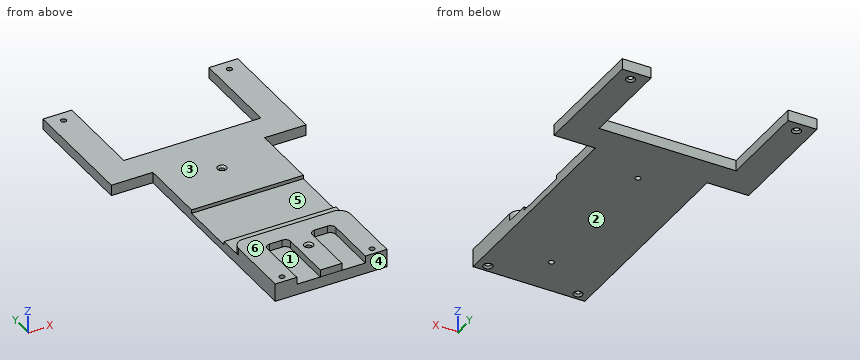
```python
from build123d import *

# Parameters (mm, degrees)
SKETCH_R        = 1.5
PAD_DEPTH       = 6
SKETCH001_R     = 1.5
PAD001_DEPTH    = 4
SKETCH002_R     = 1.5
POCKET_DEPTH    = 10
CHAMFER_SIZE    = 1
SKETCH003_W     = 100
SKETCH003_H     = 32
POCKET001_DEPTH = 2


with BuildPart() as part:
    # Sketch → Pad (new body)
    with BuildSketch(Plane.XY):
        Polygon((-38, 29), (38, 29), (38, 80), (54, 80), (54, 13), (31, 13), (31, -107), (-31, -107), (-31, 13), (-54, 13), (-54, 80), (-38, 80), align=None)
        Circle(SKETCH_R, mode=Mode.SUBTRACT)
        with Locations((0, -85)):
            Circle(SKETCH_R, mode=Mode.SUBTRACT)
        with Locations((46, 74)):
            Circle(SKETCH_R, mode=Mode.SUBTRACT)
        with Locations((-46, 74)):
            Circle(SKETCH_R, mode=Mode.SUBTRACT)
    extrude(amount=PAD_DEPTH)

    # Sketch001 (on Face18 of Pad) → Pad001 (join)
    with BuildSketch(Plane.XY.offset(6)):
        with BuildLine():
            Line((31, -71), (31, -107))
            Line((19, -107), (31, -107))
            Line((19, -78.000015), (19, -107))
            ThreePointArc((19, -78.000015), (18.12132, -75.878696), (16.000001, -75.000016))
            Line((8.999999, -75.000016), (16.000001, -75.000016))
            ThreePointArc((8.999999, -75.000016), (6.878678, -75.878697), (6, -78.000019))
            Line((6, -107.000009), (6, -78.000019))
            Line((-6, -107.000009), (6, -107.000009))
            Line((-6, -78.000019), (-6, -107.000009))
            ThreePointArc((-6, -78.000019), (-6.878676, -75.878693), (-8.999999, -75.000009))
            Line((-16.000001, -75.000009), (-8.999999, -75.000009))
            ThreePointArc((-16.000001, -75.000009), (-18.12132, -75.878689), (-19, -78.000009))
            Line((-19, -107), (-19, -78.000009))
            Line((-31, -107), (-19, -107))
            Line((-31, -107), (-31, -71))
            ThreePointArc((-25, -65), (-29.242641, -66.757359), (-31, -71))
            Line((-25, -65), (25, -65))
            ThreePointArc((31, -71), (29.242641, -66.757359), (25, -65))
        make_face()
        with Locations((0, -85)):
            Circle(SKETCH001_R, mode=Mode.SUBTRACT)
    extrude(amount=PAD001_DEPTH)

    # Sketch002 (on Face30 of Pad001) → Pocket (cut)
    with BuildSketch(Plane.XY.offset(10)):
        with Locations((-25, -103)):
            Circle(SKETCH002_R)
        with Locations((25, -103)):
            Circle(SKETCH002_R)
    extrude(amount=-POCKET_DEPTH, mode=Mode.SUBTRACT)

    # Chamfer
    chamfer_edges = [part.edges().sort_by_distance(p)[0] for p in [
        (23.5, -103, 0),
        (-26.5, -103, 0),
        (-47.5, 74, 0),
        (44.5, 74, 0),
        (-1.5, -85, 10),
        (-1.5, 0, 6),
    ]]
    chamfer(chamfer_edges, length=CHAMFER_SIZE)

    # Sketch003 (on Face21 of Chamfer) → Pocket001 (cut)
    with BuildSketch(Plane.XY.offset(6)):
        with Locations((0, -41)):
            Rectangle(SKETCH003_W, SKETCH003_H)
    extrude(amount=-POCKET001_DEPTH, mode=Mode.SUBTRACT)


solid = part.part
```
Work out the finished part from the listing and answer in its coordinate system (mm). Face numbers are marked on the shaded views. A direction names the side the tool comes from. Give positions to 0.01 mm unless a question says otherwise; leave off trailing zeros. Order: outer loops, then holes, each group sorted by start corner. A loop starts at its lowest first (then second) coordinate and runs counter-clockwise, first axis right, second up.
1. The mould has two halves that part along Y. Classify the marked faces 4, 5 and 6: released by +Y, released by -Y, zero draft, split by the parting line, or undercut.
Result sheet:
face 4: released by -Y
face 5: undercut
face 6: zero draft
2. Each of these flat-tipped pins is pushed along its axis until it touches: P1, Ø2, axis at x = 7.5, z = 9, coming from the +Y side; P2, Ø1.8, axis at x = -46, y = 74, coming from the -Z side; P3, Ø2, axis at y = -91.5, z = 7, coming from the +X side; P4, Ø2, axis at y = -99, z = 8.5, coming from the -X side. Where does it stop, or does it pass through?
Result sheet:
P1: stops at y = -65
P2: passes through
P3: stops at x = 31
P4: stops at x = -31
3. For the marked faces 1, 2 and 3, determine the directions among +Z, -Z, +X, -X, +Y, -Y from which every point of the face is accessible in a straight line to the end or side of a thin tool.
Result sheet:
face 1: +Z, -Y
face 2: -Z, +X, -X, +Y, -Y
face 3: +Z, +X, -X, +Y
4. Section B-B, the plane y = -22 is taken. Determine the outline of the cut face in (x, z).
Result sheet:
outline: (-31, 0) - (31, 0) - (31, 6) - (-31, 6) - close
5. Straight lines are drawn through the part: L1, parallel to Y at x = 25, z = 5.25; L2, parallel to Y at x = -46, z = 4.6; L3, parallel to Y at x = -8.5, z = 5.75. For each, find the intervals that lie inside material, in ascending order.
Result sheet:
L1: y = -107 to -104.5, -101.5 to -57, -25 to 29
L2: y = 13 to 72.5, 75.5 to 80
L3: y = -107 to -57, -25 to 29
6. Section A-A, the plane y = 66.5 is taken. Determine the outline of the cut face in (x, z), and give its area (3 significant figures).
Result sheet:
outline: (-54, 0) - (-38, 0) - (-38, 6) - (-54, 6) - close; (38, 0) - (54, 0) - (54, 6) - (38, 6) - close
area: 192 mm2
